Here's the drawing with two shaded views (mm, measured from the low corner). I have some questions. Give positions to 0.01 mm unless a question says otherwise; leave off trailing zeros. Loops run counter-clockwise (first coordinate to the right, second up) from the corner with the lowest first, then second, coordinate; pieces in that order, holes last.
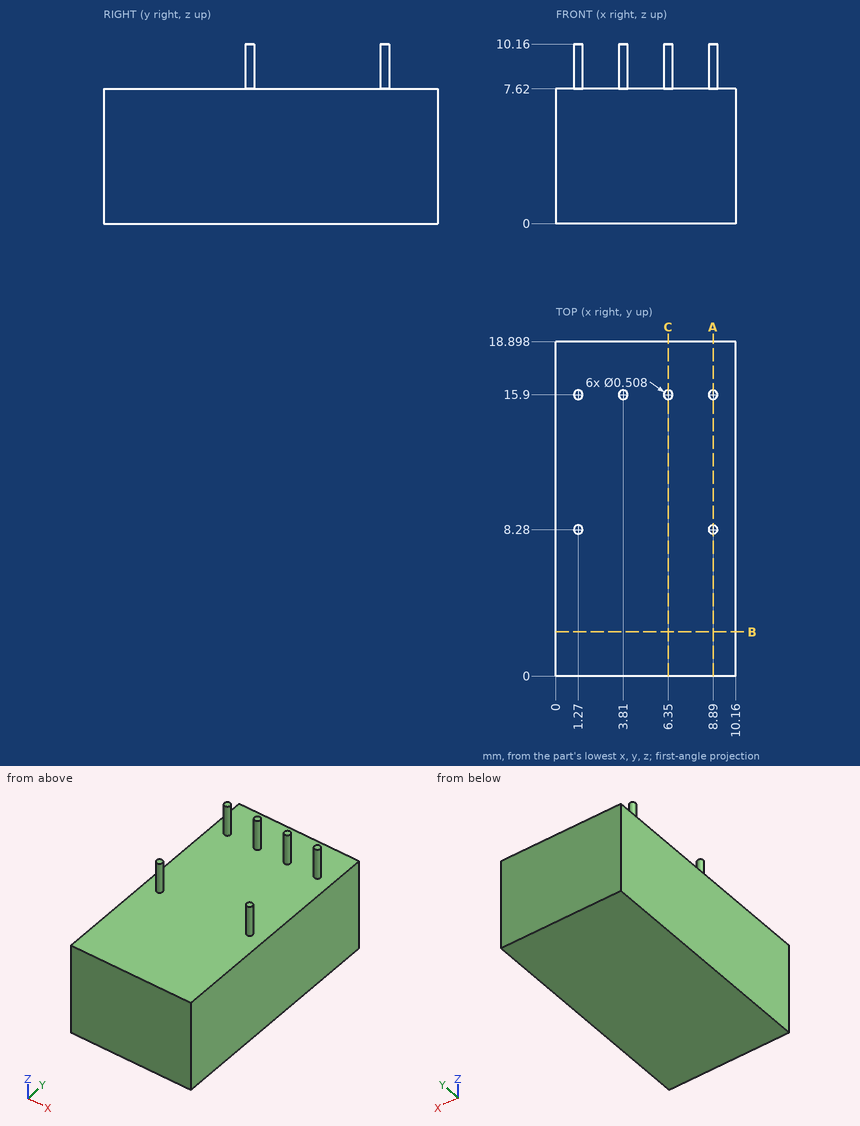
(1) Suppose I cut it at B-B on y = 2.5. List the corners of the cut face in (x, z) for me, plus the area to 3 significant figures.
Returned:
outline: (0, 0) - (10.16, 0) - (10.16, 7.62) - (0, 7.62) - close
area: 77.4 mm2
(2) Will this pin go through, and if not, where does the flat tip stop? P1, Ø1.5, axis at x = 9, z = 2.5, coming from the -Y side.
Returned:
P1: stops at y = 0
(3) Suppose I cut it at C-C on x = 6.35. List the corners of the cut face in (y, z) for me (1 decimal).
Returned:
outline: (0, 0) - (18.9, 0) - (18.9, 7.6) - (16.2, 7.6) - (16.2, 10.2) - (15.6, 10.2) - (15.6, 7.6) - (0, 7.6) - close
(4) Please list where this line runs through material, in increasing order: probe 1 along Z at (x, y) = (8.25, 17.25).
Returned:
probe 1: z = 0 to 7.62
(5) Suppose I cut it at A-A on x = 8.89. List the corners of the cut face in (y, z) for me (1 decimal).
Returned:
outline: (0, 0) - (18.9, 0) - (18.9, 7.6) - (16.2, 7.6) - (16.2, 10.2) - (15.6, 10.2) - (15.6, 7.6) - (8.5, 7.6) - (8.5, 10.2) - (8, 10.2) - (8, 7.6) - (0, 7.6) - close
